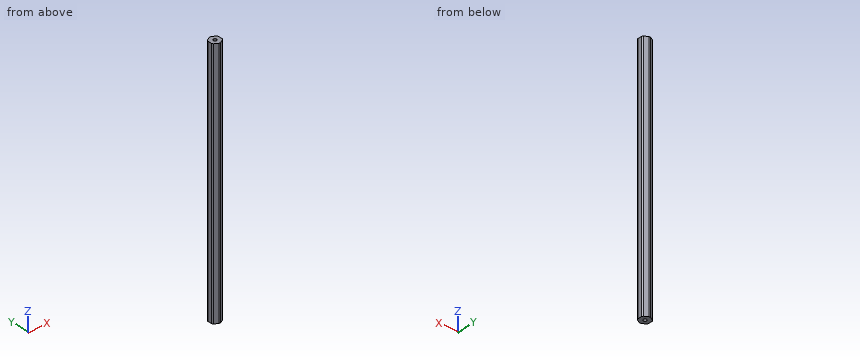
from build123d import *

# Parameters (mm, degrees)
BOSS_EXTRUDE1_DEPTH = 148.5265
SKETCH2_R           = 2.0193
CUT_EXTRUDE1_DEPTH  = 298.199999113


with BuildPart() as part:
    # Sketch1 → Boss-Extrude1 (new, symmetric)
    with BuildSketch(Plane.XY):
        with BuildLine():
            ThreePointArc((0.93173274, 6.79441227), (0, 6.858), (-0.93173274, 6.79441227))
            Line((-0.93173274, 6.79441227), (-5.41826726, 4.204110358))
            ThreePointArc((-5.41826726, 4.204110358), (-5.939202219, 3.429), (-6.35, 2.590301913))
            Line((-6.35, 2.590301913), (-6.35, -2.590301913))
            ThreePointArc((-6.35, -2.590301913), (-5.939202219, -3.429), (-5.41826726, -4.204110358))
            Line((-5.41826726, -4.204110358), (-0.93173274, -6.79441227))
            ThreePointArc((-0.93173274, -6.79441227), (0, -6.858), (0.93173274, -6.79441227))
            Line((0.93173274, -6.79441227), (5.41826726, -4.204110358))
            ThreePointArc((5.41826726, -4.204110358), (5.939202219, -3.429), (6.35, -2.590301913))
            Line((6.35, -2.590301913), (6.35, 2.590301913))
            ThreePointArc((6.35, 2.590301913), (5.939202219, 3.429), (5.41826726, 4.204110358))
            Line((5.41826726, 4.204110358), (0.93173274, 6.79441227))
        make_face()
    extrude(amount=BOSS_EXTRUDE1_DEPTH, both=True)

    # Sketch2 → Cut-Extrude1 (cut, through all)
    with BuildSketch(Plane.XY.offset(148.5265)):
        Circle(SKETCH2_R)
    extrude(amount=-CUT_EXTRUDE1_DEPTH, mode=Mode.SUBTRACT)


solid = part.part
Geometry: final body of the model. Coordinates: model frame, mm. Give positions to 0.01 mm unless a question says otherwise; leave off trailing zeros. Write each loop counter-clockwise with the first axis right and the second up, starting at its lowest first coordinate (ties: lowest second). Pieces come first, ordered by that corner, then holes. Notation, with made-up numbers: (87.5, -14.5) - (138.5, -14.5) arc R16 ccw to (138.5, 3.5) - close; hole circle Ø11 at (1, 28). An arc over 180 degrees is marked (long way). Return JSON: item names as keys, results as strings. Group by question number.
1) First-contact query: P1, Ø2.5, axis at x = 0, y = 0, coming from the -Z side; P2, Ø1.5, axis at x = -4.5, z = -92, coming from the -Y side. Flat tips, straight axial feed; report the tip coordinate or a pass-through.
2) Section A-A on z = -111.5. Return the cut outline in (x, y).
3) Line query: line 1 (Y direction, x = 0, z = -52); line 2 (X direction, y = -1.5, z = -71); line 3 (Y direction, x = 1.5, z = -85.5). Output: solid intervals per line, ascending.
Filled in:
{
 "1": {"P1": "passes through", "P2": "stops at y = -5.17"},
 "2": {"outline": "(-6.35, -2.59) arc R6.86 ccw to (-5.42, -4.2) - (-0.93, -6.79) arc R6.86 ccw to (0.93, -6.79) - (5.42, -4.2) arc R6.86 ccw to (6.35, -2.59) - (6.35, 2.59) arc R6.86 ccw to (5.42, 4.2) - (0.93, 6.79) arc R6.86 ccw to (-0.93, 6.79) - (-5.42, 4.2) arc R6.86 ccw to (-6.35, 2.59) - close; hole circle Ø4.04 at (0, 0)"},
 "3": {"line 1": "y = -6.86 to -2.02, 2.02 to 6.86", "line 2": "x = -6.35 to -1.35, 1.35 to 6.35", "line 3": "y = -6.47 to -1.35, 1.35 to 6.47"}
}
